Work out the finished part from the listing and answer in its coordinate system (mm). Face numbers are marked on the shaded views. A direction names the side the tool comes from. Give positions to 0.01 mm unless a question says otherwise; leave off trailing zeros. Order: outer loops, then holes, each group sorted by start corner. A loop starts at its lowest first (then second) coordinate and runs counter-clockwise, first axis right, second up. Notation, with made-up numbers: M 20,42 L 73,42 A26 cw 73,64 Z; hole C -13.75,0 d8. An arc over 180 degrees is marked long. One line per item, written item: value.
from build123d import *

# Parameters (mm, degrees)
SKETCH1_W                      = 50
SKETCH1_H                      = 30
BASE_FLANGE1_DEPTH             = 1
EDGE_FLANGE1_STRIP_W           = 8
EDGE_FLANGE1_STRIP_H           = 1
EDGE_FLANGE1_STRIP_CUT_DEPTH   = 30
EDGE_FLANGE1_STRIP_2_W         = 8
EDGE_FLANGE1_STRIP_2_H         = 1
EDGE_FLANGE1_STRIP_CUT_2_DEPTH = 30
EDGE_FLANGE1_DEPTH             = 30
EDGE_FLANGE1_BEND_DEPTH        = 30
EDGE_FLANGE2_STRIP_W           = 5.4732
EDGE_FLANGE2_STRIP_H           = 1
EDGE_FLANGE2_STRIP_CUT_DEPTH   = 30
EDGE_FLANGE2_STRIP_2_W         = 5.4732
EDGE_FLANGE2_STRIP_2_H         = 1
EDGE_FLANGE2_STRIP_CUT_2_DEPTH = 30
EDGE_FLANGE2_DEPTH             = 30
EDGE_FLANGE2_BEND_DEPTH        = 30
BREAK_CORNER1_START            = 20
BREAK_CORNER1_DEPTH            = 1
CUT_EXTRUDE1_DEPTH             = 10
SKETCH25_R                     = 2.5
CUT_EXTRUDE2_DEPTH             = 10
EDGE_FLANGE3_DEPTH             = 34
EDGE_FLANGE4_DEPTH             = 6
EDGE_FLANGE4_START             = -1
EDGE_FLANGE4_PROFILE_R         = 2.5
EDGE_FLANGE4_FLAT_DEPTH        = 1


# Read off the part's stored shape, not the designer's step: Break-Corner1
# Sheet-metal steps are written as plain solids
with BuildPart() as part:
    # Sketch1 → Base-Flange1 (new body)
    with BuildSketch(Plane(origin=(0, 0, 0), x_dir=(1, 0, 0), z_dir=(0, 1, 0))):
        Rectangle(SKETCH1_W, SKETCH1_H)
    extrude(amount=BASE_FLANGE1_DEPTH)

    # Edge-Flange1 strip (across the edge) → Edge-Flange1 strip cut (cut)
    with BuildSketch(Plane(origin=(25, 1, 15), x_dir=(-1, 0, 0), z_dir=(0, 0, -1))):
        with Locations((-1, -0.5)):
            Rectangle(EDGE_FLANGE1_STRIP_W, EDGE_FLANGE1_STRIP_H)
    extrude(amount=EDGE_FLANGE1_STRIP_CUT_DEPTH, mode=Mode.SUBTRACT)

    # Edge-Flange1 strip 2 (across the edge) → Edge-Flange1 strip cut 2 (cut)
    with BuildSketch(Plane(origin=(-25, 1, -15), x_dir=(1, 0, 0), z_dir=(0, 0, 1))):
        with Locations((-1, -0.5)):
            Rectangle(EDGE_FLANGE1_STRIP_2_W, EDGE_FLANGE1_STRIP_2_H)
    extrude(amount=EDGE_FLANGE1_STRIP_CUT_2_DEPTH, mode=Mode.SUBTRACT)

    # Edge-Flange1 section (across the edge) → Edge-Flange1 (add)
    with BuildSketch(Plane(origin=(25, 1, 15), x_dir=(-1, 0, 0), z_dir=(0, 0, -1))):
        with BuildLine():
            Line((0, 2), (0, 19))
            Line((0, 19), (1, 19))
            Line((1, 19), (1, 2))
            ThreePointArc((1, 2), (1.585786438, 0.585786438), (3, 0))
            Line((3, 0), (3, -1))
            ThreePointArc((3, -1), (0.878679656, -0.121320344), (0, 2))
        make_face()
    extrude(amount=EDGE_FLANGE1_DEPTH)

    # Edge-Flange1 section 2 (across the edge) → Edge-Flange1 bend (add)
    with BuildSketch(Plane(origin=(-25, 1, -15), x_dir=(1, 0, 0), z_dir=(0, 0, 1))):
        with BuildLine():
            Line((0, 2), (0, 19))
            Line((0, 19), (1, 19))
            Line((1, 19), (1, 2))
            ThreePointArc((1, 2), (1.585786438, 0.585786438), (3, 0))
            Line((3, 0), (3, -1))
            ThreePointArc((3, -1), (0.878679656, -0.121320344), (0, 2))
        make_face()
    extrude(amount=EDGE_FLANGE1_BEND_DEPTH)

    # Edge-Flange2 strip (across the edge) → Edge-Flange2 strip cut (cut)
    with BuildSketch(Plane(origin=(25, 20, -15), x_dir=(0, -1, 0), z_dir=(0, 0, 1))):
        with Locations((-2, -0.5)):
            Rectangle(EDGE_FLANGE2_STRIP_W, EDGE_FLANGE2_STRIP_H)
    extrude(amount=EDGE_FLANGE2_STRIP_CUT_DEPTH, mode=Mode.SUBTRACT)

    # Edge-Flange2 strip 2 (across the edge) → Edge-Flange2 strip cut 2 (cut)
    with BuildSketch(Plane(origin=(-25, 20, 15), x_dir=(0, -1, 0), z_dir=(0, 0, -1))):
        with Locations((-2, -0.5)):
            Rectangle(EDGE_FLANGE2_STRIP_2_W, EDGE_FLANGE2_STRIP_2_H)
    extrude(amount=EDGE_FLANGE2_STRIP_CUT_2_DEPTH, mode=Mode.SUBTRACT)

    # Edge-Flange2 section (across the edge) → Edge-Flange2 (add)
    with BuildSketch(Plane(origin=(25, 20, -15), x_dir=(0, -1, 0), z_dir=(0, 0, 1))):
        with BuildLine():
            Line((-1, 0.7366), (-1, 16.5))
            Line((-1, 16.5), (0, 16.5))
            Line((0, 16.5), (0, 0.7366))
            ThreePointArc((0, 0.7366), (0.215745145, 0.215745145), (0.7366, 0))
            Line((0.7366, 0), (0.7366, -1))
            ThreePointArc((0.7366, -1), (-0.491361636, -0.491361636), (-1, 0.7366))
        make_face()
    extrude(amount=EDGE_FLANGE2_DEPTH)

    # Edge-Flange2 section 2 (across the edge) → Edge-Flange2 bend (add)
    with BuildSketch(Plane(origin=(-25, 20, 15), x_dir=(0, -1, 0), z_dir=(0, 0, -1))):
        with BuildLine():
            Line((-1, 0.7366), (-1, 16.5))
            Line((-1, 16.5), (0, 16.5))
            Line((0, 16.5), (0, 0.7366))
            ThreePointArc((0, 0.7366), (0.215745145, 0.215745145), (0.7366, 0))
            Line((0.7366, 0), (0.7366, -1))
            ThreePointArc((0.7366, -1), (-0.491361636, -0.491361636), (-1, 0.7366))
        make_face()
    extrude(amount=EDGE_FLANGE2_BEND_DEPTH)

    # Break-Corner1 outline → Break-Corner1 (cut)
    with BuildSketch(Plane(origin=(0, 0, 0), x_dir=(1, 0, 0), z_dir=(0, 1, 0)).offset(BREAK_CORNER1_START)):
        with BuildLine():
            Line((41.5, -15), (41.5, -9))
            ThreePointArc((41.5, -9), (39.742640687, -13.242640687), (35.5, -15))
            Line((35.5, -15), (41.5, -15))
        make_face()
        with BuildLine():
            ThreePointArc((35.5, 15), (39.742640687, 13.242640687), (41.5, 9))
            Line((41.5, 9), (41.5, 15))
            Line((41.5, 15), (35.5, 15))
        make_face()
        with BuildLine():
            Line((-41.5, -15), (-35.5, -15))
            ThreePointArc((-35.5, -15), (-39.742640687, -13.242640687), (-41.5, -9))
            Line((-41.5, -9), (-41.5, -15))
        make_face()
        with BuildLine():
            Line((-41.5, 15), (-41.5, 9))
            ThreePointArc((-41.5, 9), (-39.742640687, 13.242640687), (-35.5, 15))
            Line((-35.5, 15), (-41.5, 15))
        make_face()
    extrude(amount=BREAK_CORNER1_DEPTH, mode=Mode.SUBTRACT)

    # Sketch24 → Cut-Extrude1 (cut)
    with BuildSketch(Plane(origin=(0, 1, 0), x_dir=(1, 0, 0), z_dir=(0, 1, 0))):
        with BuildLine():
            Line((-9, 8), (9, 8))
            ThreePointArc((9, 8), (17, 0), (9, -8))
            Line((9, -8), (-9, -8))
            ThreePointArc((-9, -8), (-17, 0), (-9, 8))
        make_face()
    extrude(amount=-CUT_EXTRUDE1_DEPTH, mode=Mode.SUBTRACT)

    # Sketch25 → Cut-Extrude2 (cut)
    with BuildSketch(Plane(origin=(0, 21, 0), x_dir=(1, 0, 0), z_dir=(0, 1, 0))):
        with Locations(Location((-35.5, 9, 0), (0, 0, 270))):
            Circle(SKETCH25_R)
        with Locations(Location((-35.5, -9, 0), (0, 0, 270))):
            Circle(SKETCH25_R)
    cut_extrude2 = extrude(amount=-CUT_EXTRUDE2_DEPTH, mode=Mode.SUBTRACT)

    # Mirror1: Cut-Extrude2 across plane
    add(cut_extrude2.mirror(Plane(origin=(0, 0, 0), x_dir=(0, 0, 1), z_dir=(1, 0, 0))), mode=Mode.SUBTRACT)

    # Edge-Flange3 section (across the edge) → Edge-Flange3 (add)
    with BuildSketch(Plane(origin=(17, 0, 15.7366), x_dir=(0, 0, -1), z_dir=(-1, 0, 0))):
        with BuildLine():
            Line((-1, 0.7366), (-1, 14))
            Line((-1, 14), (0, 14))
            Line((0, 14), (0, 0.7366))
            ThreePointArc((0, 0.7366), (0.215745145, 0.215745145), (0.7366, 0))
            Line((0.7366, 0), (0.7366, -1))
            ThreePointArc((0.7366, -1), (-0.491361636, -0.491361636), (-1, 0.7366))
        make_face()
    extrude(amount=EDGE_FLANGE3_DEPTH)

    # Edge-Flange4 bend section (across the edge) → Edge-Flange4 (add)
    with BuildSketch(Plane(origin=(-17.7366, -8, 16.7366), x_dir=(1, 0, 0), z_dir=(0, -1, 0))):
        with BuildLine():
            Line((-1, 0.7366), (0, 0.7366))
            ThreePointArc((0, 0.7366), (0.215745145, 0.215745145), (0.7366, 0))
            Line((0.7366, 0), (0.7366, -1))
            ThreePointArc((0.7366, -1), (-0.491361636, -0.491361636), (-1, 0.7366))
        make_face()
    edge_flange4 = extrude(amount=EDGE_FLANGE4_DEPTH)

    # Edge-Flange4 profile (on flange) → Edge-Flange4 flat (add)
    with BuildSketch(Plane(origin=(-17.7366, 0, 16.7366), x_dir=(0, 1, 0), z_dir=(1, 0, 0)).offset(EDGE_FLANGE4_START)):
        with BuildLine():
            ThreePointArc((-23, 14), (-28, 9), (-23, 4))
            Line((-23, 4), (-14, 4))
            Line((-14, 4), (-14, 0.7366))
            Line((-14, 0.7366), (-8, 0.7366))
            Line((-8, 0.7366), (-8, 14))
            Line((-8, 14), (-14, 14))
            Line((-14, 14), (-23, 14))
        make_face()
        with Locations((-23, 9)):
            Circle(EDGE_FLANGE4_PROFILE_R, mode=Mode.SUBTRACT)
    edge_flange4_flat = extrude(amount=EDGE_FLANGE4_FLAT_DEPTH)

    # Mirror2: Edge-Flange4, Edge-Flange4 flat across plane
    add(edge_flange4.mirror(Plane(origin=(0, 0, 0), x_dir=(0, 0, 1), z_dir=(1, 0, 0))))
    add(edge_flange4_flat.mirror(Plane(origin=(0, 0, 0), x_dir=(0, 0, 1), z_dir=(1, 0, 0))))


solid = part.part
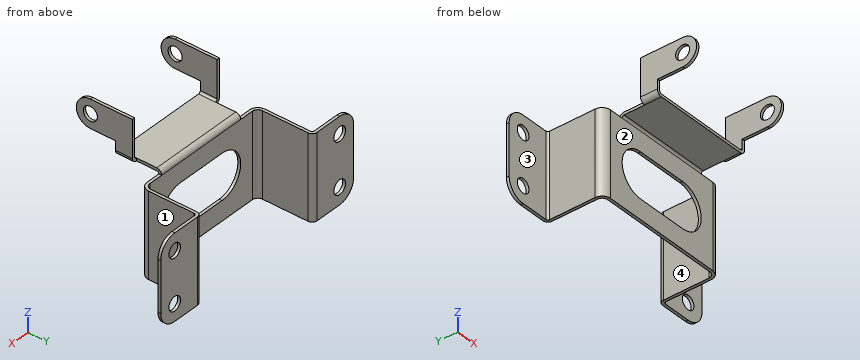
(1) Section B-B, the plane y = 9 is taken. Give the vertices of the cut face in (x, z).
Findings:
outline: M -25,-15 L -24,-15 L -24,15 L -25,15 Z; M 24,-15 L 25,-15 L 25,15 L 24,15 Z
(2) Find the intervals of material crossed by probe 1 along X at (y, z) = (18.5, -7); probe 2 along Z at (x, y) = (-18, -23); probe 3 along Y at (x, z) = (-1, -13), in increasing order. Write a range as from..to.
Findings:
probe 1: x = -25..-24, 24..25
probe 2: z = 20.74..23.24, 28.24..30.74
probe 3: y = 0..1
(3) Section A-A, the plane z = 0 is taken. Give the vertices of the cut face in (x, y).
Findings:
outline: M -41.5,20 L -25.74,20 A0.74 cw -25,19.26 L -25,3 A3 ccw -22,0 L -17,0 L -17,1 L -22,1 A2 cw -24,3 L -24,19.26 A1.74 ccw -25.74,21 L -41.5,21 Z; M 17,0 L 22,0 A3 ccw 25,3 L 25,19.26 A0.74 cw 25.74,20 L 41.5,20 L 41.5,21 L 25.74,21 A1.74 ccw 24,19.26 L 24,3 A2 cw 22,1 L 17,1 Z
(4) Which of the six approach directions +Z, -Z, +X, -X, +Y, -Y give full straight-line access (tool end or side, diameter ignored) to the marked faces 1, 2, 3 and 4?
Findings:
face 1: +Z, -Z, +X, -Y
face 2: -Z, +X, -X, -Y
face 3: +Z, -Z, -X, -Y
face 4: +Z, -Z, +Y
(5) Section C-C, the plane x = 15.5 is taken. Give the vertices of the cut face in (y, z).
Findings:
outline: M -14,15.74 L -0.74,15.74 A0.74 cw 0,15 L 0,4.66 L 1,4.66 L 1,15 A1.74 ccw -0.74,16.74 L -14,16.74 Z; M 0,-15 L 1,-15 L 1,-4.66 L 0,-4.66 Z
(6) Given P1, Ø8, axis at y = 12, z = 4, coming from the +X side; P2, Ø10.5, axis at y = -17, z = 27.5, coming from the +X side; P3, Ø13, axis at y = 11.5, z = 0, coming from the -X side; P4, Ø9, axis at x = 7, z = 0, coming from the -Y side, each flat-ended and moving along its own axis, determine where each tip first touches the part or whether it passes through.
Findings:
P1: stops at x = 25
P2: stops at x = 18.74
P3: stops at x = -25
P4: passes through
(7) Section D-D, the plane z = 13.5 is taken. Give the vertices of the cut face in (x, y), then the cut area to 3 significant figures.
Findings:
outline: M -39.47,20 L -25.74,20 A0.74 cw -25,19.26 L -25,3 A3 ccw -22,0 L 22,0 A3 ccw 25,3 L 25,19.26 A0.74 cw 25.74,20 L 39.47,20 L 39.47,21 L 25.74,21 A1.74 ccw 24,19.26 L 24,3 A2 cw 22,1 L -22,1 A2 cw -24,3 L -24,19.26 A1.74 ccw -25.74,21 L -39.47,21 Z
area: 116 mm^2
